For this review, take the finished solid that the model builds, in its own axes (mm). A direction names the side the tool comes from. Coordinates: 2 decimals unless noted, no trailing zeros. Loops run counter-clockwise (first coordinate to the right, second up) from the corner with the lowest first, then second, coordinate; pieces in that order, holes last.
```python
from build123d import *

# Parameters (mm, degrees)
SKETCH1_W           = 50
SKETCH1_H           = 50
SKETCH1_R           = 24
BOSS_EXTRUDE1_DEPTH = 15.5
CHAMFER1_SIZE       = 3
SKETCH4_W           = 50
SKETCH4_H           = 50
SKETCH4_W_2         = 48
SKETCH4_H_2         = 48
BOSS_EXTRUDE2_DEPTH = 15.5
SKETCH5_R           = 2.75
CUT_EXTRUDE1_DEPTH  = 3
FILLET1_R           = 4
SKETCH6_R           = 12.5
BOSS_EXTRUDE5_DEPTH = 1
SKETCH7_R           = 2
CUT_EXTRUDE2_DEPTH  = 21
CHAMFER3_SIZE       = 0.75
SKETCH9_W           = 3
SKETCH9_H           = 24
BOSS_EXTRUDE6_DEPTH = 1
CIRPATTERN1_COUNT   = 3


# Some blends are built 0.0001 mm under size
with BuildPart() as part:
    # Sketch1 → Boss-Extrude1 (new body)
    with BuildSketch(Plane(origin=(0, 0, 0), x_dir=(1, 0, 0), z_dir=(0, 1, 0))):
        Rectangle(SKETCH1_W, SKETCH1_H)
        with Locations(Location((0, 0, 0), (0, 0, 270))):
            Circle(SKETCH1_R, mode=Mode.SUBTRACT)
    extrude(amount=BOSS_EXTRUDE1_DEPTH)

    # Chamfer1
    # the kernel refuses this chamfer: 3 mm, written as the material it takes off along each edge
    with BuildSketch(Plane(origin=(0, 15.5, 0), x_dir=(0, 0, 1), z_dir=(-1, 0, 0))) as chamfer1_piece_1:
        Polygon((24, -CHAMFER1_SIZE), (24 + CHAMFER1_SIZE, 0), (24, 0), align=None)
    revolve(axis=Axis((0, 15.5, 0), (0, 1, 0)), mode=Mode.SUBTRACT)

    # Sketch4 → Boss-Extrude2 (add)
    with BuildSketch(Plane(origin=(0, 15.5, 0), x_dir=(1, 0, 0), z_dir=(0, 1, 0))):
        Rectangle(SKETCH4_W, SKETCH4_H)
        Rectangle(SKETCH4_W_2, SKETCH4_H_2, mode=Mode.SUBTRACT)
    extrude(amount=-BOSS_EXTRUDE2_DEPTH)

    # Sketch5 → Cut-Extrude1 (cut)
    with BuildSketch(Plane(origin=(0, 15.5, 0), x_dir=(1, 0, 0), z_dir=(0, 1, 0))):
        with Locations(Location((-19.25, 19.25, 0), (0, 0, 270))):
            Circle(SKETCH5_R)
        with Locations(Location((19.25, 19.25, 0), (0, 0, 270))):
            Circle(SKETCH5_R)
        with Locations(Location((19.25, -19.25, 0), (0, 0, 270))):
            Circle(SKETCH5_R)
        with Locations(Location((-19.25, -19.25, 0), (0, 0, 270))):
            Circle(SKETCH5_R)
    extrude(amount=-CUT_EXTRUDE1_DEPTH, mode=Mode.SUBTRACT)

    # Fillet1
    fillet1_edges = [part.edges().sort_by_distance(p)[0] for p in [
        (-25, 7.75, -25),
        (25, 7.75, -25),
        (25, 7.75, 25),
        (-25, 7.75, 25),
    ]]
    fillet(fillet1_edges, radius=FILLET1_R)

    # Sketch7 → Cut-Extrude2 (cut)
    with BuildSketch(Plane(origin=(0, 12.5, 0), x_dir=(1, 0, 0), z_dir=(0, 1, 0))):
        with Locations(Location((-19.25, 19.25, 0), (0, 0, 270))):
            Circle(SKETCH7_R)
        with Locations(Location((-19.25, -19.25, 0), (0, 0, 270))):
            Circle(SKETCH7_R)
        with Locations(Location((19.25, -19.25, 0), (0, 0, 270))):
            Circle(SKETCH7_R)
        with Locations(Location((19.25, 19.25, 0), (0, 0, 270))):
            Circle(SKETCH7_R)
    extrude(amount=-CUT_EXTRUDE2_DEPTH, mode=Mode.SUBTRACT)

    # Chamfer3
    chamfer3_edges = [part.edges().sort_by_distance(p)[0] for p in [
        (-19.25, 12.5, -21.25),
        (-19.25, 12.5, 17.25),
        (19.25, 12.5, 17.25),
        (19.25, 12.5, -21.25),
    ]]
    chamfer(chamfer3_edges, length=CHAMFER3_SIZE - 0.0001)  # a hair under: the kernel refuses the full size



with BuildPart() as body_2:
    # Sketch6 → Boss-Extrude5 (new body)
    with BuildSketch(Plane(origin=(0, 0, 0), x_dir=(1, 0, 0), z_dir=(0, 1, 0))):
        with Locations(Location((0, 0, 0), (0, 0, 270))):
            Circle(SKETCH6_R)
    extrude(amount=BOSS_EXTRUDE5_DEPTH)


with BuildPart() as part_1:
    add(part.part)

    add(body_2.part)  # Boss-Extrude6 merges body 2
    # Sketch9 → Boss-Extrude6 (add)
    with BuildSketch(Plane.XZ):
        with Locations((0, 12.5)):
            Rectangle(SKETCH9_W, SKETCH9_H)
    boss_extrude6 = extrude(amount=-BOSS_EXTRUDE6_DEPTH)

    # CirPattern1: Boss-Extrude6 ×3 about axis
    cirpattern1_axis = Axis((0, 0, 0), (0, 1, 0))
    for i in range(1, CIRPATTERN1_COUNT):
        add(boss_extrude6.rotate(cirpattern1_axis, i * 360 / CIRPATTERN1_COUNT))


solid = part_1.part
```
Q1. Wall thickness on probe 1 along Z at (x, y) = (-19.25, 14.8); probe 2 along Z at (x, y) = (19.25, 13.1); probe 3 along X at (y, z) = (4, -19.25): over which ranges is each line inside the solid? List them lowest first.
Q2. Machinability: for faces 4 (the face through (16.426, 0.493, -7.751)), 5 (the face through (0, 8, -25)), 6 (the face through (1, 1, 0)), which of the approach directions +Z, -Z, +X, -X, +Y, -Y give a long, thin tool a straight path to every point of the face, cutting with its end or side? Answer none if there is none.
Q3. Consider section B-B (z = -19.25). Count the separate pieces of the cut face and the enclosed holes in it, then the cut area to 3 significant figures.
Q4. For pin 1 Ø4.5 at (x, z) = (-19.25, -19.25) entering from +Y; pin 2 Ø12 at (x, z) = (5, 15) entering from +Y; pin 3 Ø10 at (x, z) = (-7.5, -18) entering from +Y, all flat-tipped, find the tip position at first contact; note any pin that passes through.
Q5. The part is to be moulded in two halves that separate along Z. For faces 1 (the face through (23.797, 7.858, 23.859)), 2 (the face through (-17.267, 5.957, -19.51)), 3 (the face through (0, 0, 0)), say which applies: +Z half, -Z half, draft (parallel to the pull), parting line (faces both ways), or undercut.
Q6. Consider section A-A (y = 4). State the section outline as (x, z) points.
Model answer:
1. probe 1: z = -25 to -22, 22 to 25
1. probe 2: z = -25 to -22, -16.5 to -15.32, 15.32 to 16.5, 22 to 25
1. probe 3: x = -25 to -21.25, -17.25 to -14.33, 14.33 to 17.25, 21.25 to 25
2. face 4: +Y, -Y
2. face 5: -Z, +X, -X, +Y, -Y
2. face 6: +Y
3. separate pieces: 4
3. enclosed holes: 0
3. area: 186 mm2
4. pin 1: stops at y = 12
4. pin 2: stops at y = 1
4. pin 3: stops at y = 13
5. face 1: +Z half
5. face 2: undercut
5. face 3: draft
6. outline: (-25, -21) arc R4 ccw to (-21, -25) - (21, -25) arc R4 ccw to (25, -21) - (25, 21) arc R4 ccw to (21, 25) - (-21, 25) arc R4 ccw to (-25, 21) - close; hole circle Ø48 at (0, 0); hole circle Ø4 at (-19.25, -19.25); hole circle Ø4 at (-19.25, 19.25); hole circle Ø4 at (19.25, -19.25); hole circle Ø4 at (19.25, 19.25)
